from build123d import *

# Parameters (mm, degrees)
BOSS_EXTRUDE1_DEPTH = 50
SKETCH2_R           = 1.5
BOSS_EXTRUDE2_DEPTH = 8
SKETCH3_R           = 1.5
CUT_EXTRUDE1_DEPTH  = 10
CHAMFER1_SIZE       = 0.3


with BuildPart() as part:
    # Sketch1 → Boss-Extrude1 (new body)
    with BuildSketch(Plane(origin=(0, 0, 0), x_dir=(0, 0, -1), z_dir=(1, 0, 0))):
        Polygon((0, 3.175426481), (-2.75, 1.58771324), (-2.75, -1.58771324), (0, -3.175426481), (2.75, -1.58771324), (2.75, 1.58771324), align=None)
    extrude(amount=BOSS_EXTRUDE1_DEPTH)

    # Sketch2 → Boss-Extrude2 (add)
    with BuildSketch(Plane(origin=(50, 0, 0), x_dir=(0, 0, -1), z_dir=(1, 0, 0))):
        Circle(SKETCH2_R)
    extrude(amount=BOSS_EXTRUDE2_DEPTH)

    # Sketch3 → Cut-Extrude1 (cut)
    with BuildSketch(Plane.ZY):
        Circle(SKETCH3_R)
    extrude(amount=-CUT_EXTRUDE1_DEPTH, mode=Mode.SUBTRACT)

    # Sketch4 → Cut-Revolve1 (revolve, cut)
    with BuildSketch(Plane(origin=(0, 0, 0), x_dir=(1, 0, 0), z_dir=(0, 1, 0))):
        Polygon((0, 10.219809024), (4.392081913, 10.219809024), (0, 2.6125), align=None)
        Polygon((50, 2.6125), (50, 10.219809024), (45.607918087, 10.219809024), align=None)
    revolve(axis=Axis((0, 0, 0), (-1, 0, 0)), mode=Mode.SUBTRACT)

    # Chamfer1
    chamfer1_edges = [part.edges().sort_by_distance(p)[0] for p in [
        (58, 0, 1.5),
    ]]
    chamfer(chamfer1_edges, length=CHAMFER1_SIZE)


solid = part.part
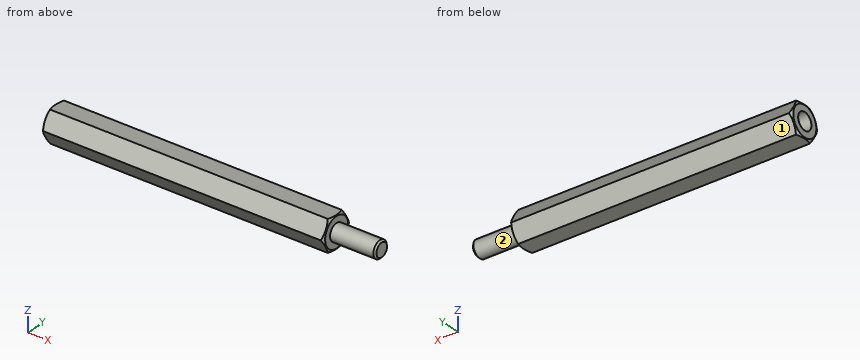
Could you check a few things on this model? Use its own coordinates, in mm. Face numbers are marked on the shaded views. A direction names the side the tool comes from. Give positions to 0.01 mm unless a question says otherwise; leave off trailing zeros. Order: outer loops, then holes, each group sorted by start corner. A loop starts at its lowest first (then second) coordinate and runs counter-clockwise, first axis right, second up. Notation, with made-up numbers: (26, -35.75) -> (53, -35.75) arc R33 cw to (53, 1.25) -> close; hole circle Ø2 at (16, -21). An arc over 180 degrees is marked (long way). Return JSON: item names as keys, results as strings.
1. On a 3-axis mill with a long thin cutter (end or side, diameter ignored), from which of +Z, -Z, +X, -X, +Y, -Y can I reach the whole of each face in a straight line? I mean the marked faces 1 and 2. Say none if no direction works.
Answer list:
{"face 1": "-Z, +X, -X, +Y", "face 2": "+X"}
2. For pin 1 Ø1 at (y, z) = (-2, 2) entering from -X; pin 2 Ø2 at (x, z) = (42, 1.5) entering from -Y, each with a flat end and sliding along its axis, tell me the tip position at first contact or that it passes through.
Answer list:
{"pin 1": "stops at x = 0", "pin 2": "stops at y = -2.89"}
3. I need wall thicknesses on line 1 (Y direction, x = 4.25, z = 0); line 2 (X direction, y = 1.75, z = -1.4); line 3 (X direction, y = 1, z = -0.35). Which ranges of each line are inside material? Lowest first, please. Write a range as from..to.
Answer list:
{"line 1": "y = -3.18..-1.5, 1.5..3.18", "line 2": "x = 0..50", "line 3": "x = 10..58"}
4. Imagine slicing it at A-A on y = 0. List the corners of the cut face in (x, z) for me.
Answer list:
{"outline": "(0, -2.61) -> (0.08, -2.75) -> (49.92, -2.75) -> (50, -2.61) -> (50, -1.5) -> (57.7, -1.5) -> (58, -1.2) -> (58, 1.2) -> (57.7, 1.5) -> (50, 1.5) -> (50, 2.61) -> (49.92, 2.75) -> (0.08, 2.75) -> (0, 2.61) -> (0, 1.5) -> (10, 1.5) -> (10, -1.5) -> (0, -1.5) -> close"}
5. Imagine slicing it at B-B on x = 32. List the corners of the cut face in (y, z) for me.
Answer list:
{"outline": "(-3.18, 0) -> (-1.59, -2.75) -> (1.59, -2.75) -> (3.18, 0) -> (1.59, 2.75) -> (-1.59, 2.75) -> close"}
